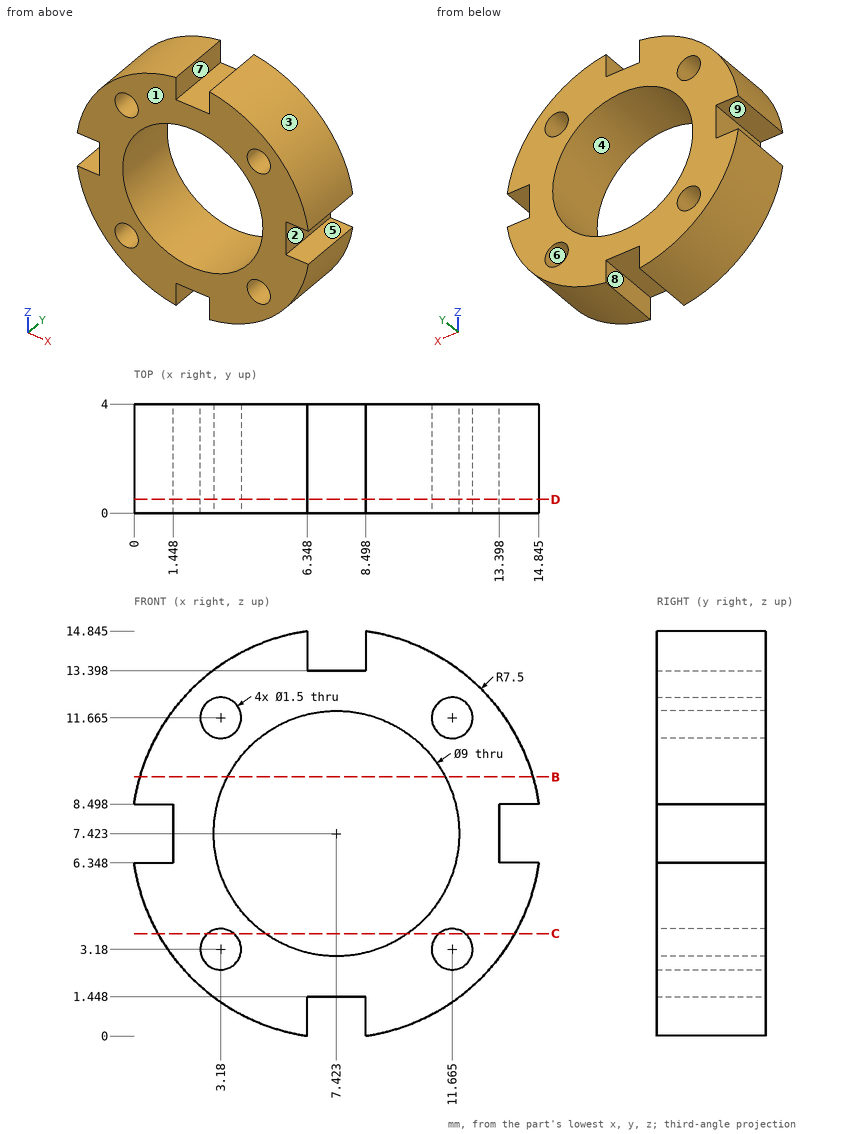
Could you check a few things on this drawing? It's one solid part, dimensions in mm from its lowest x, y, z. A direction names the side the tool comes from. Coordinates: 2 decimals unless noted, no trailing zeros. Write each loop counter-clockwise with the first axis right and the second up, starting at its lowest first coordinate (ties: lowest second). Pieces come first, ordered by that corner, then holes. Notation, with made-up numbers: (87, 0.5) - (143, 0.5) arc R28 cw to (143, 20.5) - close; hole circle Ø1 at (51, -36.75). An arc over 180 degrees is marked (long way). Put each result on its own line as item: value. Start each with the question number.
Q1. Thinking about a two-plate mould opening in Z: for the marked faces 1, 2, 3 and 4, which applies, pulls with the +Z half, pulls with the -Z half, needs draft (parallel to the pull), parting line crosses it, or undercut?
Q2. I want a section at B-B on z = 9.5. Write out the boundary of the cut face in (x, y) (1 decimal).
Q3. I'm going to push flat-ended pins straight in: P1, Ø0.6, axis at y = 1, z = 7.5, coming from the +X side; P2, Ø1.6, axis at x = 1, y = 2.5, coming from the +Z side (1 decimal); P3, Ø1.1, axis at y = 1.5, z = 7.5, coming from the -X side. Where does each tip first touch, or does it pass through?
Q4. Which directions (+Z, -Z, +X, -X, +Y, -Y) give clear straight access to the entire face, cutting with the end or side of a thin tool? Please do the marked faces 5, 6, 7, 8 and 9.
Q5. Please list where these lines run through material, in increasing order: L1, parallel to X at y = 1.2, z = 3.5 (1 decimal); L2, parallel to Z at x = 11.25, y = 3 (1 decimal); L3, parallel to X at y = 2.85, z = 7.5.
Q6. I want a section at C-C on z = 3.75. Write out the boundary of the cut face in (x, y).
Q7. I want a section at D-D on y = 0.5. Count the separate pieces of the cut face and the enclosed holes in it.
Checks:
1. face 1: needs draft
1. face 2: undercut
1. face 3: pulls with the +Z half
1. face 4: undercut
2. outline: (0.2, 0) - (3.4, 0) - (3.4, 4) - (0.2, 4) - close; (11.4, 0) - (14.6, 0) - (14.6, 4) - (11.4, 4) - close
3. P1: x = 13.4
3. P2: z = 12.4
3. P3: x = 1.45
4. face 5: +X, +Y, -Y
4. face 6: +Y, -Y
4. face 7: +Z, +Y, -Y
4. face 8: -Z, +Y, -Y
4. face 9: -X, +Y, -Y
5. L1: 1 to 2.5, 3.9 to 5.2, 9.6 to 11, 12.3 to 13.8
5. L2: 1 to 2.6, 3.8 to 5.1, 9.8 to 11, 12.3 to 13.9
5. L3: 1.45 to 2.92, 11.92 to 13.4
6. outline: (0.88, 0) - (2.69, 0) - (2.69, 4) - (0.88, 4) - close; (3.67, 0) - (4.82, 0) - (4.82, 4) - (3.67, 4) - close; (10.02, 0) - (11.18, 0) - (11.18, 4) - (10.02, 4) - close; (12.15, 0) - (13.96, 0) - (13.96, 4) - (12.15, 4) - close
7. separate pieces: 1
7. enclosed holes: 5
